from build123d import *

# Parameters (mm, degrees)
F0_W        = 74.5
F0_H        = 21.5
F0_R        = 10.55
F1_DEPTH    = 40
F2_R        = 5
F7_W        = 18.8593324274
F7_H        = 1.088095014
F8_DEPTH    = 5
F9_T1_DEPTH = 34.4293351412
F10_R       = 3.825
F11_DEPTH   = 25
F12_R       = 3.825
F13_DEPTH   = 25


# Not quite as in the source:
# - a fillet or chamfer that OpenCascade refuses, or shapes differently, is made with other operations: its cross-section is extruded or revolved along the edge and cut away or added


with BuildPart() as f1:
    # F0 (on Top) → F1 (new body)
    with BuildSketch(Plane.XY):
        Rectangle(F0_W, F0_H)
        with Locations((-24.6931102476, 0)):
            Circle(F0_R, mode=Mode.SUBTRACT)
        with BuildLine():
            ThreePointArc((35.3068897524, 0), (24.7568897524, -10.55), (14.2068897524, 0))
            ThreePointArc((14.2068897524, 0), (24.7568897524, 10.55), (35.3068897524, 0))
        make_face(mode=Mode.SUBTRACT)
        with Locations((-24.6931102476, 0)):
            Circle(F0_R)
        with BuildLine():
            ThreePointArc((35.3068897524, 0), (24.7568897524, 10.55), (14.2068897524, 0))
            ThreePointArc((14.2068897524, 0), (24.7568897524, -10.55), (35.3068897524, 0))
        make_face()
    extrude(amount=F1_DEPTH)

    # F2
    f2_edges = [f1.edges().sort_by_distance(p)[0] for p in [
        (-37.25, -10.75, 20),
        (37.25, -10.75, 20),
        (-37.25, 10.75, 20),
        (37.25, 10.75, 20),
    ]]
    fillet(f2_edges, radius=F2_R)

    # F3 (on Front) → F4 (revolve, cut)
    with BuildSketch(Plane.XZ):
        with BuildLine():
            Line((-35.1722761989, 0), (-28.4331102476, 0))
            Line((-28.4331102476, 0), (-28.4331102476, 10.0509282202))
            ThreePointArc((-28.4331102476, 10.0509282202), (-32.7146634372, 5.6369418244), (-35.1722761989, 0))
        make_face()
    revolve(axis=Axis((-24.6931102476, 0, 9.2185929652), (0, 0, 1)), mode=Mode.SUBTRACT)

    # F5 (on Front) → F6 (revolve, cut)
    with BuildSketch(Plane.XZ):
        with BuildLine():
            Line((28.4479595721, 9.307410568), (28.4479595721, 0))
            Line((28.4479595721, 0), (35.168658942, 0))
            ThreePointArc((35.168658942, 0), (32.9055101663, 5.445972629), (28.4479595721, 9.307410568))
        make_face()
    revolve(axis=Axis((24.7338861227, 0, 7.0413234644), (0, 0, 1)), mode=Mode.SUBTRACT)

    # F7 (on face) → F8 (join)
    with BuildSketch(Plane.XZ.offset(10.75)):
        with Locations((0.5516856909, 0.544047507)):
            Rectangle(F7_W, F7_H)
    extrude(amount=F8_DEPTH)

    # F9: fillet of radius 5 on 1 edges, made by hand

    # F9_s2 → F9_t1 (cut)
    with BuildSketch(Plane.YZ.offset(-16.6629818797)):
        with BuildLine():
            ThreePointArc((-12.6359994572, 1.088095014), (-14.2853137193, 0.8082393407), (-15.75, 0))
            Line((-15.75, 0), (-15.75, 1.088095014))
            Line((-15.75, 1.088095014), (-12.6359994572, 1.088095014))
        make_face()
    extrude(amount=F9_T1_DEPTH, mode=Mode.SUBTRACT)

    # F10 (on Top) → F11 (cut)
    with BuildSketch(Plane.XY):
        with Locations((-24.7297555931, 0)):
            Circle(F10_R)
    extrude(amount=F11_DEPTH, mode=Mode.SUBTRACT)

    # F12 (on Top) → F13 (cut)
    with BuildSketch(Plane.XY):
        with Locations((24.8167866624, 0)):
            Circle(F12_R)
    extrude(amount=F13_DEPTH, mode=Mode.SUBTRACT)


solid = f1.part
CAD build for the part. Positions are in the model's coordinates, mm. A direction names the side the tool comes from. Give positions to 0.01 mm unless a question says otherwise; leave off trailing zeros. Order: outer loops, then holes, each group sorted by start corner. A loop starts at its lowest first (then second) coordinate and runs counter-clockwise, first axis right, second up. Notation, with made-up numbers: (-31, 88.25) -> (23, 88.25) arc R17 cw to (23, 97.25) -> close; hole circle Ø7 at (37, 60.5). An arc over 180 degrees is marked (long way). Return JSON: item names as keys, results as strings.
Q1. Which spindle directions (+Z, -Z, +X, -X, +Y, -Y) get a long thin tool onto all of the face, cutting with end or side? Do faces 4 (the face through (0, -12, 1.088)), 5 (the face through (25, 0, 25)), 6 (the face through (35.82, 9.25, 20.28)). Say none if no direction does.
Working result:
{"face 4": "+Z, +X, -X, -Y", "face 5": "-Z", "face 6": "+Z, -Z, +X, +Y"}
Q2. Mould opens along Y. For faces 1 (the face through (37.25, 0, 20)), 2 (the face through (-25, 0, 25)), 3 (the face through (35.75, -9.32, 20.28)) say: pulls with the +Y half, pulls with the -Y half, needs draft (parallel to the pull), parting line crosses it, or undercut.
Working result:
{"face 1": "needs draft", "face 2": "undercut", "face 3": "pulls with the -Y half"}
Q3. Saw through at C-C (z = 6). Count the separate pieces of the cut face and the enclosed holes in it, then the cut area to 3 significant figures.
Working result:
{"separate pieces": "1", "enclosed holes": "2", "area": "1,200 mm²"}
Q4. Drill centre lines: line 1 (X direction, y = 0, z = 13); line 2 (X direction, y = -7, z = 3); line 3 (Y direction, x = -19.5, z = 15). Where is each one in solid material? Low to high.
Working result:
{"line 1": "-37.25 to -28.55, -20.9 to 20.99, 28.64 to 37.25", "line 2": "-37.09 to -31.08, -18.31 to 18.23, 31.24 to 37.09", "line 3": "-10.75 to 10.75"}
Q5. Flat gauge pins, fed straight in: pin 1 (4 mm diameter, centred on x = 12, z = 7, fed in from -Y); pin 2 (1 mm diameter, centred on y = -12, z = 28, fed in from -X); pin 3 (6 mm diameter, centred on x = 22.5, y = -11.5, fed in from -Z); pin 4 (1.2 mm diameter, centred on y = -13, z = 0.5, fed in from +X). Where does each tip first touch, or does it go through?
Working result:
{"pin 1": "y = -10.75", "pin 2": "through", "pin 3": "z = 0", "pin 4": "x = 9.98"}
Q6. Saw through at A-A (z = 20.5). Write the cut outline in (x, y) (3 decimals).
Working result:
{"outline": "(-37.25, -5.75) arc R5 ccw to (-32.25, -10.75) -> (32.25, -10.75) arc R5 ccw to (37.25, -5.75) -> (37.25, 5.75) arc R5 ccw to (32.25, 10.75) -> (-32.25, 10.75) arc R5 ccw to (-37.25, 5.75) -> close; hole circle Ø7.65 at (-24.73, 0); hole circle Ø7.65 at (24.817, 0)"}
Q7. Saw through at B-B (z = 37). Write the cut outline in (x, y).
Working result:
{"outline": "(-37.25, -5.75) arc R5 ccw to (-32.25, -10.75) -> (32.25, -10.75) arc R5 ccw to (37.25, -5.75) -> (37.25, 5.75) arc R5 ccw to (32.25, 10.75) -> (-32.25, 10.75) arc R5 ccw to (-37.25, 5.75) -> close"}
